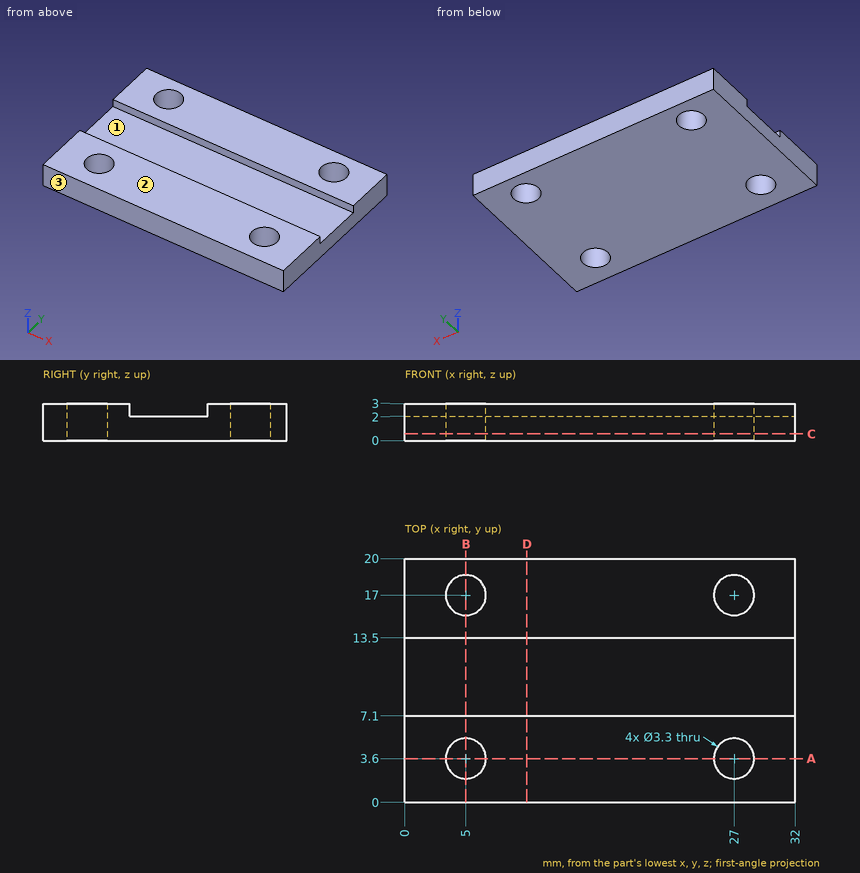
Input: dimensioned drawing with shaded views. Units: mm. Origin: part minimum x, y, z. Coordinates: 2 decimals unless noted, no trailing zeros. Loops run counter-clockwise (first coordinate to the right, second up) from the corner with the lowest first, then second, coordinate; pieces in that order, holes last. Notation, with made-up numbers: M -35,15 L -30,15 A21 ccw -30,37 Z; hole C 68.5,50 d4. An arc over 180 degrees is marked long. Put each result on its own line as item: value.
(1) Cut plane B-B on x = 5. Return the cut outline in (y, z), then the cut area to 3 significant figures.
Answer sheet:
outline: M 0,0 L 1.95,0 L 1.95,3 L 0,3 Z; M 5.25,0 L 15.35,0 L 15.35,3 L 13.5,3 L 13.5,2 L 7.1,2 L 7.1,3 L 5.25,3 Z; M 18.65,0 L 20,0 L 20,3 L 18.65,3 Z
area: 33.8 mm^2
(2) Material intervals for probe 1 along Y at (x, z) = (5, 2.1); probe 2 along Y at (x, z) = (27, 0.6); probe 3 along Z at (x, y) = (11, 7.25), sorted ascending.
Answer sheet:
probe 1: y = 0 to 1.95, 5.25 to 7.1, 13.5 to 15.35, 18.65 to 20
probe 2: y = 0 to 1.95, 5.25 to 15.35, 18.65 to 20
probe 3: z = 0 to 2
(3) Cut plane D-D on x = 10. Return the cut outline in (y, z).
Answer sheet:
outline: M 0,0 L 20,0 L 20,3 L 13.5,3 L 13.5,2 L 7.1,2 L 7.1,3 L 0,3 Z
(4) Draft query along Y for the marked faces 1, 2 and 3. Return one class per face: pulls with the +Y half, pulls with the -Y half, needs draft (parallel to the pull), parting line crosses it, or undercut.
Answer sheet:
face 1: undercut
face 2: needs draft
face 3: pulls with the -Y half
(5) Cut plane A-A on y = 3.6. Return the cut outline in (x, z), then the cut area to 3 significant figures.
Answer sheet:
outline: M 0,0 L 3.35,0 L 3.35,3 L 0,3 Z; M 6.65,0 L 25.35,0 L 25.35,3 L 6.65,3 Z; M 28.65,0 L 32,0 L 32,3 L 28.65,3 Z
area: 76.2 mm^2
(6) Cut plane C-C on z = 0.55. Return the cut outline in (x, y), then the cut area to 3 significant figures.
Answer sheet:
outline: M 0,0 L 32,0 L 32,20 L 0,20 Z; hole C 5,3.6 d3.3; hole C 5,17 d3.3; hole C 27,3.6 d3.3; hole C 27,17 d3.3
area: 606 mm^2
(7) First-contact query: pin 1 (3 mm diameter, centred on x = 12.5, y = 11.5, fed in from +Z). Flat tip, straight axial feed; report the tip coordinate or a pass-through.
Answer sheet:
pin 1: stops at z = 2
